Check sheet for the modelled part. Datum: model origin and axes. Units: mm. Face numbers are marked on the shaded views. A direction names the side the tool comes from. Round coordinates to 2 decimals unless told otherwise and drop trailing zeros. Write each loop counter-clockwise with the first axis right and the second up, starting at its lowest first coordinate (ties: lowest second). Pieces come first, ordered by that corner, then holes.
Item 1: Release check for a two-part mould opening along X. For the marked faces 1, 2, 3 and 4 record: +X half, -X half, draft (parallel to the pull), parting line (faces both ways), or undercut.
Item 2: Cross-section at D-D on z = 13.75. Enter the section's corners in (x, y).
Item 3: Cross-section at B-B on x = -10.5. Enter the section's corners in (y, z).
Item 4: Cross-section at C-C on z = 4.25. Enter the section's corners in (x, y), plus the area to 3 significant figures.
Item 5: Cross-section at A-A on y = -2.75. Enter the section's corners in (x, z), plus the area to 3 significant figures.
Item 6: Go/stop test with a flat-tipped pin: pin 1 Ø0.8 at (x, y) = (14.5, -2) entering from +Z. Record where the tip stops, or that it passes through.
Item 7: Tool access check on the marked faces 5 and 6. Record the directions out of +Z, -Z, +X, -X, +Y, -Y that give a thin tool (end or side, any length) a straight path to the whole face; none if there is none.
Item 8: Material ranges on line 1 (X direction, y = -12.25, z = 4.75); line 2 (X direction, y = 1.5, z = 11), recorded low to high.
from build123d import *

# Parameters (mm, degrees)
F0_W     = 30
F0_H     = 30
F0_W_2   = 28
F0_H_2   = 28
F1_DEPTH = 15
F2_W     = 10
F2_H     = 5
F3_DEPTH = 25


with BuildPart() as f1:
    # F0 (on Top) → F1 (new body)
    with BuildSketch(Plane.XY):
        Rectangle(F0_W, F0_H)
        Rectangle(F0_W_2, F0_H_2, mode=Mode.SUBTRACT)
    extrude(amount=F1_DEPTH)

    # F2 (on face) → F3 (cut)
    with BuildSketch(Plane.YZ.offset(15)):
        with Locations((0, 17.5)):
            Rectangle(F2_W, F2_H)
        with Locations((0, 12.5)):
            Rectangle(F2_W, F2_H)
    extrude(amount=-F3_DEPTH, mode=Mode.SUBTRACT)


solid = f1.part
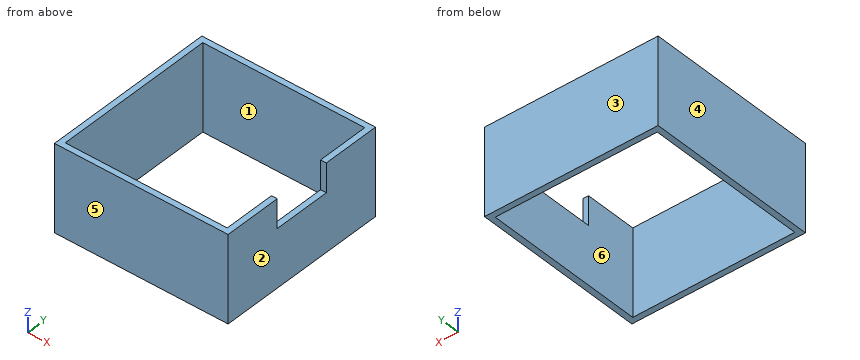
Response values:
1. face 1: undercut
1. face 2: +X half
1. face 3: draft
1. face 4: -X half
2. outline: (-15, -15) - (15, -15) - (15, -5) - (14, -5) - (14, -14) - (-14, -14) - (-14, 14) - (14, 14) - (14, 5) - (15, 5) - (15, 15) - (-15, 15) - close
3. outline: (-15, 0) - (-14, 0) - (-14, 15) - (-15, 15) - close; (14, 0) - (15, 0) - (15, 15) - (14, 15) - close
4. outline: (-15, -15) - (15, -15) - (15, 15) - (-15, 15) - close; hole (-14, -14) - (14, -14) - (14, 14) - (-14, 14) - close
4. area: 116 mm2
5. outline: (-15, 0) - (-14, 0) - (-14, 15) - (-15, 15) - close; (14, 0) - (15, 0) - (15, 10) - (14, 10) - close
5. area: 25.0 mm2
6. pin 1: stops at z = 10
7. face 5: +Z, -Z, +X, -X, -Y
7. face 6: +Z, -Z
8. line 1: x = -15 to -14, 14 to 15
8. line 2: x = -15 to -14
